```python
from build123d import *

# Parameters (mm, degrees)
EXTRUDE_20_DEPTH           = 20
CUT_EXTRUDE_5_DEPTH        = 59.172158289
CUT_EXTRUDE_5_DEPTH_BACK   = 59.172158289
SKETCH_5_R                 = 2.75
CUT_EXTRUDE_5_4_3_DEPTH    = 4.3
CUT_EXTRUDE_5_2_DEPTH      = 59.172158289
CUT_EXTRUDE_5_2_DEPTH_BACK = 59.172158289
SKETCH_5_3_R               = 2.75
CUT_EXTRUDE_5_4_3_2_DEPTH  = 4.3


with BuildPart() as part:
    # Профиль_скобы_6мм → Печатный_корпус_20мм (new body)
    with BuildSketch(Plane.XY):
        Polygon((6.15, -22), (12.15, -22), (12.15, -6), (50, -6), (50, 0), (6.15, 0), align=None)
    extrude(amount=EXTRUDE_20_DEPTH)

    # Sketch 5 → Cut-Extrude 5 (cut, two sides: drawn at the far end of the back side and taken through both)
    with BuildSketch(Plane(origin=(0, 0, 0), x_dir=(1, 0, 0), z_dir=(0, 1, 0)).offset(-CUT_EXTRUDE_5_DEPTH_BACK)):
        with Locations(Location((32, -10, 0), (0, 0, 270))):
            Circle(SKETCH_5_R)
    extrude(amount=CUT_EXTRUDE_5_DEPTH + CUT_EXTRUDE_5_DEPTH_BACK, mode=Mode.SUBTRACT)

    # Sketch 5 2 → Cut-Extrude 5_4_3 (cut)
    with BuildSketch(Plane.XZ.offset(6)):
        Polygon((32, 14.792007234), (36.15, 12.396003617), (36.15, 7.603996383), (32, 5.207992766), (27.85, 7.603996383), (27.85, 12.396003617), align=None)
    extrude(amount=-CUT_EXTRUDE_5_4_3_DEPTH, mode=Mode.SUBTRACT)

    # Sketch 5 3 → Cut-Extrude 5 2 (cut, two sides: drawn at the far end of the back side and taken through both)
    with BuildSketch(Plane(origin=(0, 0, 0), x_dir=(0, 0, -1), z_dir=(1, 0, 0)).offset(-CUT_EXTRUDE_5_2_DEPTH_BACK)):
        with Locations(Location((-10, -12, 0), (0, 0, 180))):
            Circle(SKETCH_5_3_R)
    extrude(amount=CUT_EXTRUDE_5_2_DEPTH + CUT_EXTRUDE_5_2_DEPTH_BACK, mode=Mode.SUBTRACT)

    # Sketch 5 4 → Cut-Extrude 5_4_3 2 (cut)
    with BuildSketch(Plane(origin=(12.15, 0, 0), x_dir=(0, 0, -1), z_dir=(1, 0, 0))):
        Polygon((-10, -7.207992766), (-14.15, -9.603996383), (-14.15, -14.396003617), (-10, -16.792007234), (-5.85, -14.396003617), (-5.85, -9.603996383), align=None)
    extrude(amount=-CUT_EXTRUDE_5_4_3_2_DEPTH, mode=Mode.SUBTRACT)


solid = part.part
```
CAD build for the part. Positions are in the model's coordinates, mm. A direction names the side the tool comes from. Coordinates: 2 decimals unless noted, no trailing zeros. Order: outer loops, then holes, each group sorted by start corner. A loop starts at its lowest first (then second) coordinate and runs counter-clockwise, first axis right, second up.
(1) Saw through at C-C, the plane y = -12. Write the cut outline in (x, z).
Solution:
outline: (6.15, 0) - (12.15, 0) - (12.15, 5.85) - (7.85, 5.85) - (7.85, 7.25) - (6.15, 7.25) - close; (6.15, 12.75) - (7.85, 12.75) - (7.85, 14.15) - (12.15, 14.15) - (12.15, 20) - (6.15, 20) - close
(2) Pin check, flat tips, straight feed: pin 1 Ø4 at (y, z) = (-9.5, 12) entering from +X; pin 2 Ø2 at (y, z) = (-15, 10) entering from +X; pin 3 Ø1 at (x, z) = (32, 4) entering from -Y. Stop position of each tip, or through.
Solution:
pin 1: stops at x = 12.15
pin 2: stops at x = 7.85
pin 3: stops at y = -6
(3) Drill centre lines: L1, parallel to X at y = -5, z = 11.5; L2, parallel to Y at x = 7.4, z = 10; L3, parallel to X at y = -0.6, z = 10. Where is each one in solid material? Low to high.
Solution:
L1: x = 6.15 to 27.85, 36.15 to 50
L2: y = -22 to -14.75, -9.25 to 0
L3: x = 6.15 to 29.25, 34.75 to 50
(4) Saw through at B-B, the plane y = -5. Write the cut outline in (x, z).
Solution:
outline: (6.15, 0) - (50, 0) - (50, 20) - (6.15, 20) - close; hole (27.85, 7.6) - (32, 5.21) - (36.15, 7.6) - (36.15, 12.4) - (32, 14.79) - (27.85, 12.4) - close
(5) Mould opens along X. For faces 1 (the face through (29.95, -3.88, 6.39)), 2 (the face through (7.85, -12, 13)), 3 (the face through (23, -4, 20)) say: released by +X, released by -X, zero draft, split by the parting line, or undercut.
Solution:
face 1: undercut
face 2: released by +X
face 3: zero draft
(6) Saw through at A-A, the plane z = 9.5. Write the cut outline in (x, y).
Solution:
outline: (6.15, -22) - (12.15, -22) - (12.15, -16.5) - (7.85, -16.5) - (7.85, -14.7) - (6.15, -14.7) - close; (6.15, -9.3) - (7.85, -9.3) - (7.85, -7.5) - (12.15, -7.5) - (12.15, -6) - (27.85, -6) - (27.85, -1.7) - (29.3, -1.7) - (29.3, 0) - (6.15, 0) - close; (34.7, -1.7) - (36.15, -1.7) - (36.15, -6) - (50, -6) - (50, 0) - (34.7, 0) - close
(7) Which spindle directions (+Z, -Z, +X, -X, +Y, -Y) get a long thin tool onto all of the face, cutting with end or side? Do faces 4 (the face through (6.99, -14.32, 11.48)), 5 (the face through (10.03, -15.58, 12.1)), 6 (the face through (34.1, -3.88, 6.42)), 7 (the face through (27, -6, 10)), 8 (the face through (50, -3, 10)). Say none if no direction does.
Solution:
face 4: +X, -X
face 5: +X
face 6: -Y
face 7: +Z, -Z, +X, -Y
face 8: +Z, -Z, +X, +Y, -Y
(8) Saw through at D-D, the plane z = 3.75. Write the cut outline in (x, y).
Solution:
outline: (6.15, -22) - (12.15, -22) - (12.15, -6) - (50, -6) - (50, 0) - (6.15, 0) - close
